```python
from build123d import *

# Parameters (mm, degrees)
SKETCH2_W           = 127
SKETCH2_H           = 76.2
SKETCH2_R           = 10.5
SKETCH2_R_2         = 1.5
BOSS_EXTRUDE1_DEPTH = 6.35
SKETCH3_R           = 4
BOSS_EXTRUDE2_DEPTH = 6.35
LPATTERN1_COUNT     = 2
LPATTERN1_PITCH     = 38.1
BOSS_EXTRUDE3_START = -38.1
SKETCH4_R           = 5
BOSS_EXTRUDE3_DEPTH = 3.175


with BuildPart() as part:
    # Sketch2 → Boss-Extrude1 (new body)
    with BuildSketch(Plane(origin=(0, 0, 0), x_dir=(1, 0, 0), z_dir=(0, 1, 0))):
        Rectangle(SKETCH2_W, SKETCH2_H)
        with Locations(Location((-40.1, 0, 0), (0, 0, 270))):
            Circle(SKETCH2_R, mode=Mode.SUBTRACT)
        with Locations(Location((11.3, 10, 0), (0, 0, 270))):
            Circle(SKETCH2_R_2, mode=Mode.SUBTRACT)
        with Locations(Location((-57.25, 17.15, 0), (0, 0, 270))):
            Circle(SKETCH2_R_2, mode=Mode.SUBTRACT)
        with Locations(Location((-57.25, -17.15, 0), (0, 0, 90))):
            Circle(SKETCH2_R_2, mode=Mode.SUBTRACT)
        with Locations(Location((-11.7, 10, 0), (0, 0, 90))):
            Circle(SKETCH2_R_2, mode=Mode.SUBTRACT)
        with Locations(Location((-22.95, -17.15, 0), (0, 0, 270))):
            Circle(SKETCH2_R_2, mode=Mode.SUBTRACT)
        with Locations(Location((-22.95, 17.15, 0), (0, 0, 90))):
            Circle(SKETCH2_R_2, mode=Mode.SUBTRACT)
        with Locations(Location((11.3, -10, 0), (0, 0, 90))):
            Circle(SKETCH2_R_2, mode=Mode.SUBTRACT)
        with Locations(Location((-11.7, -10, 0), (0, 0, 270))):
            Circle(SKETCH2_R_2, mode=Mode.SUBTRACT)
    extrude(amount=BOSS_EXTRUDE1_DEPTH)

    # Sketch3 → Boss-Extrude2 (add)
    with BuildSketch(Plane(origin=(63.5, 0, 0), x_dir=(0, 0, -1), z_dir=(1, 0, 0))):
        Polygon((-38.1, 0), (38.1, 0), (38.1, 25.4), (21.451862696, 25.4), (9.5, 6.35), (-9.5, 6.35), (-21.165528848, 25.4), (-38.1, 25.4), align=None)
        with Locations((-25.4, 15.875)):
            Circle(SKETCH3_R, mode=Mode.SUBTRACT)
        with Locations((25.4, 15.875)):
            Circle(SKETCH3_R, mode=Mode.SUBTRACT)
    boss_extrude2 = extrude(amount=-BOSS_EXTRUDE2_DEPTH)

    # LPattern1: Boss-Extrude2 ×2
    with Locations(*[(-i * LPATTERN1_PITCH, 0, 0) for i in range(1, LPATTERN1_COUNT)]):
        add(boss_extrude2)

    # Sketch4 → Boss-Extrude3 (add, symmetric)
    with BuildSketch(Plane(origin=(0, 0, -38.1), x_dir=(-1, 0, 0), z_dir=(0, 0, -1)).offset(BOSS_EXTRUDE3_START)):
        with BuildLine():
            Line((-63.5, 0), (-20.400000165, 0))
            Line((-20.400000165, 0), (-38.766166206, -39.799546929))
            ThreePointArc((-38.766166206, -39.799546929), (-42.640726317, -44.24435534), (-48.3, -45.9))
            Line((-48.3, -45.9), (-53, -45.9))
            ThreePointArc((-53, -45.9), (-60.424621202, -42.824621202), (-63.5, -35.4))
            Line((-63.5, -35.4), (-63.5, 0))
        make_face()
        with Locations((-48.3, -35.4)):
            Circle(SKETCH4_R, mode=Mode.SUBTRACT)
    extrude(amount=BOSS_EXTRUDE3_DEPTH, both=True)


solid = part.part
```
The model under review builds one solid part; all positions refer to its coordinate system, in mm. A direction names the side the tool comes from. Give positions to 0.01 mm unless a question says otherwise; leave off trailing zeros. Write each loop counter-clockwise with the first axis right and the second up, starting at its lowest first coordinate (ties: lowest second). Pieces come first, ordered by that corner, then holes. Notation, with made-up numbers: (69, -33) - (94, -33) arc R25 cw to (94, -18) - close; hole circle Ø7 at (-6, 3.5). An arc over 180 degrees is marked (long way). Answer in a Markdown table with one row per item. Add a question column.
1. Insertion check: P1, Ø4, axis at x = 31.5, z = -15, coming from the -Y side; P2, Ø3.5, axis at x = -57.25, z = 17.15, coming from the +Y side; P3, Ø5.5, axis at y = 11.5, z = -21.5, coming from the -X side. Each pin has a flat end and moves straight along its axis. Give the tip position at first contact, or say it passes through.
2. We need section D-D on z = -26.5. Write out the cut boundary in (x, y), then the cut area to 3 significant figures.
3. Draft analysis for pull direction Z (two halves, no side actions). For faces 1 (the flat face through (19.05, 12, 27)), 2 (the cylindrical face through (-12.6, 3.1, 8.8)), state which applies: +Z half, -Z half, draft (parallel to the pull), parting line (faces both ways), or undercut.
4. We need section B-B on y = -37.5. Write out the cut boundary in (x, z) (3 decimals).
5. We need section C-C on x = 34.5. Write out the cut boundary in (y, z) (3 decimals).
6. We need section A-A on z = -17.15. Write out the cut boundary in (x, y), then the cut area to 3 significant figures.
7. Tool access review of faces 3 (the flat face through (22, 25.4, -30)), 4 (the flat face through (22.27, 16.01, -15.56)), 5 (the flat face through (57.15, 12, -27)), 6 (the cylindrical face through (60.369, 17.076, 21.585)), 7 (the flat face through (19.05, 12, -27)): name each direction out of +Z, -Z, +X, -X, +Y, -Y from which nothing blocks a thin tool from reaching the whole face with its end or side.
8. Wall thickness on line 1 along X through (y, z) = (4, -17); line 2 along Y through (x, z) = (62.25, 25.4) (3 decimals); line 3 along X through (y, z) = (20.5, -32): over which ranges is each line inside the solid? List them lowest first. Write a range as [from, to].
Ans:
| question | item | result |
|---|---|---|
| 1 | P1 | stops at y = 0 |
| 1 | P2 | stops at y = 6.35 |
| 1 | P3 | stops at x = 19.05 |
| 2 | outline | (-63.5, 0) - (63.5, 0) - (63.5, 12.03) - (57.15, 12.03) - (57.15, 6.35) - (25.4, 6.35) - (25.4, 12.03) - (19.05, 12.03) - (19.05, 6.35) - (-63.5, 6.35) - close; (19.05, 19.72) - (25.4, 19.72) - (25.4, 25.4) - (19.05, 25.4) - close; (57.15, 19.72) - (63.5, 19.72) - (63.5, 25.4) - (57.15, 25.4) - close |
| 2 | area | 951 mm^2 |
| 3 | face 1 | draft |
| 3 | face 2 | undercut |
| 4 | outline | (37.705, -3.175) - (43.762, -3.175) - (43.762, 3.175) - (37.705, 3.175) - close; (52.838, -3.175) - (63.288, -3.175) - (63.288, 3.175) - (52.838, 3.175) - close |
| 5 | outline | (-30.555, -3.175) - (0, -3.175) - (0, -38.1) - (6.35, -38.1) - (6.35, 38.1) - (0, 38.1) - (0, 3.175) - (-30.555, 3.175) - close |
| 6 | outline | (-63.5, 0) - (-58.75, 0) - (-58.75, 6.35) - (-63.5, 6.35) - close; (-55.75, 0) - (-24.45, 0) - (-24.45, 6.35) - (-55.75, 6.35) - close; (-21.45, 0) - (63.5, 0) - (63.5, 18.54) - (57.15, 18.54) - (57.15, 6.35) - (25.4, 6.35) - (25.4, 18.54) - (19.05, 18.54) - (19.05, 6.35) - (-21.45, 6.35) - close |
| 6 | area | 923 mm^2 |
| 7 | face 3 | +Z, -Z, +X, -X, +Y |
| 7 | face 4 | +X, -X, +Y |
| 7 | face 5 | +Z, -Z, +Y |
| 7 | face 6 | +X, -X |
| 7 | face 7 | +Z, -Z, -X, +Y |
| 8 | line 1 | x = [-63.5, -58.74], [-55.76, -24.44], [-21.46, 63.5] |
| 8 | line 2 | y = [0, 11.875], [19.875, 25.4] |
| 8 | line 3 | x = [19.05, 25.4], [57.15, 63.5] |
